Source: CAD feature listing. Evaluate the final solid. Frame: model axes, mm. Coordinates: 2 decimals unless noted, no trailing zeros. Write each loop counter-clockwise with the first axis right and the second up, starting at its lowest first coordinate (ties: lowest second). Pieces come first, ordered by that corner, then holes. Notation, with made-up numbers: (84, -0.75) - (95, -0.75) arc R6 cw to (95, 10.25) - close; hole circle Ø11 at (-18, 55.5). An arc over 180 degrees is marked (long way). One line per question, with ' | ' between items.
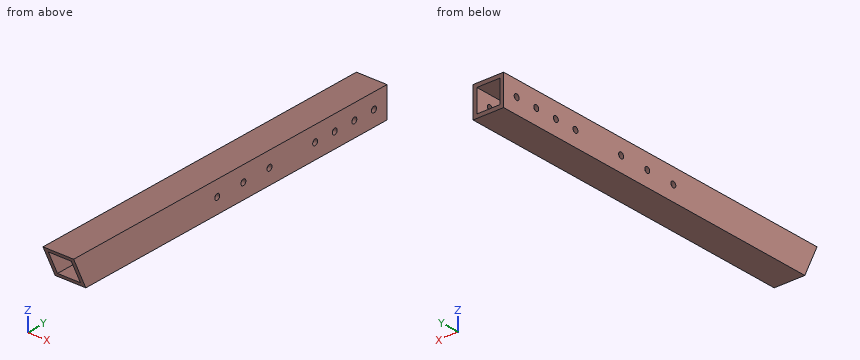
from build123d import *

# Parameters (mm, degrees)
SKETCH1_W           = 25.4
SKETCH1_H           = 25.4
SKETCH1_W_2         = 19.05
SKETCH1_H_2         = 19.05
BOSS_EXTRUDE1_DEPTH = 304.8
SKETCH2_R           = 2.413
CUT_EXTRUDE1_DEPTH  = 25.4


with BuildPart() as part:
    # Sketch1 → Boss-Extrude1 (new body)
    with BuildSketch(Plane(origin=(0, 0, 0), x_dir=(1, 0, 0), z_dir=(0, 1, 0))):
        Rectangle(SKETCH1_W, SKETCH1_H)
        Rectangle(SKETCH1_W_2, SKETCH1_H_2, mode=Mode.SUBTRACT)
    extrude(amount=BOSS_EXTRUDE1_DEPTH)

    # Sketch2 → Cut-Extrude1 (cut)
    with BuildSketch(Plane(origin=(12.7, 0, 0), x_dir=(0, 0, -1), z_dir=(1, 0, 0))):
        with Locations((0, 292.1)):
            Circle(SKETCH2_R)
        with Locations((0, 273.05)):
            Circle(SKETCH2_R)
        with Locations((0, 254)):
            Circle(SKETCH2_R)
        with Locations((0, 234.95)):
            Circle(SKETCH2_R)
        with Locations((0, 190.5)):
            Circle(SKETCH2_R)
        with Locations((0, 165.1)):
            Circle(SKETCH2_R)
        with Locations((0, 139.7)):
            Circle(SKETCH2_R)
        Polygon((-12.7, 0), (12.7, 11.844214517), (12.7, 0), align=None)
    extrude(amount=-CUT_EXTRUDE1_DEPTH, mode=Mode.SUBTRACT)


solid = part.part
Item 1: Cut plane A-A on x = 2. Return loops of the section in (y, z) (3 decimals), and give its area (3 significant figures).
Check sheet entries:
outline: (0, 12.7) - (1.481, 9.525) - (304.8, 9.525) - (304.8, 12.7) - close; (10.364, -9.525) - (11.844, -12.7) - (304.8, -12.7) - (304.8, -9.525) - close | area: 1,900 mm²
Item 2: Cut plane B-B on y = 157.5. Return loops of the section in (x, z) (3 decimals).
Check sheet entries:
outline: (-12.7, -12.7) - (12.7, -12.7) - (12.7, 12.7) - (-12.7, 12.7) - close; hole (-9.525, -9.525) - (9.525, -9.525) - (9.525, 9.525) - (-9.525, 9.525) - close
Item 3: Ray query, line 1 along X through (y, z) = (179, 0) (3 decimals); line 2 along Z through (x, y) = (12.05, 234.95). Return the intervals inside material, ascending. Write a range as [from, to].
Check sheet entries:
line 1: [-12.7, -9.525], [9.525, 12.7] | line 2: [-12.7, -2.41], [2.41, 12.7]
Item 4: Pin query (flat end, axial travel): pin 1 Ø3 at (y, z) = (292.1, 0) entering from -X; pin 2 Ø8 at (x, z) = (3.5, -6.5) entering from +Y. Return the tip coordinate at first contact, or that it passes through.
Check sheet entries:
pin 1: through | pin 2: y = 304.8
